```python
from build123d import *

# Parameters (mm, degrees)
SKETCH1_W                                       = 100
SKETCH1_H                                       = 28
BOSS_EXTRUDE1_DEPTH                             = 8
CSK_FOR_M6_FLAT_HEAD_MACHINE_SCREW1_D           = 6.6
CSK_FOR_M6_FLAT_HEAD_MACHINE_SCREW1_DEPTH       = 8
CSK_FOR_M6_FLAT_HEAD_MACHINE_SCREW1_CSINK_D     = 12.6
CSK_FOR_M6_FLAT_HEAD_MACHINE_SCREW1_CSINK_ANGLE = 90


with BuildPart() as part:
    # Sketch1 → Boss-Extrude1 (new body)
    with BuildSketch(Plane(origin=(0, 0, 0), x_dir=(1, 0, 0), z_dir=(0, 1, 0))):
        Rectangle(SKETCH1_W, SKETCH1_H)
    extrude(amount=BOSS_EXTRUDE1_DEPTH)

    # CSK for M6 Flat Head Machine Screw1
    with Locations(Plane(origin=(0, 8, 0), x_dir=(-1, 0, 0), z_dir=(0, 1, 0))):
        with Locations((-30, 0), (30, 0)):
            CounterSinkHole(CSK_FOR_M6_FLAT_HEAD_MACHINE_SCREW1_D / 2, CSK_FOR_M6_FLAT_HEAD_MACHINE_SCREW1_CSINK_D / 2, depth=CSK_FOR_M6_FLAT_HEAD_MACHINE_SCREW1_DEPTH, counter_sink_angle=CSK_FOR_M6_FLAT_HEAD_MACHINE_SCREW1_CSINK_ANGLE)


solid = part.part
```
Here's how the part is built. I have some questions about the finished solid (model axes, mm). Round coordinates to 2 decimals unless told otherwise and drop trailing zeros. Write each loop counter-clockwise with the first axis right and the second up, starting at its lowest first coordinate (ties: lowest second). Pieces come first, ordered by that corner, then holes.
Q1. If we mould it in two halves opening along Z, with no side actions, what happens to faces 1 (the flat face through (-1, 8, 0)), 2 (the conical face through (-26.71, 5.15, 1.03)), 3 (the flat face through (-1, 4, 14))? For each: +Z half, -Z half, draft (parallel to the pull), parting line (faces both ways), or undercut.
Q2. If we section it at B-B on y = 6.75: Write out the boundary of the cut face in (x, z).
Q3. Please list where these lines run through material, in increasing order: probe 1 along X at (y, z) = (3.1, 0); probe 2 along Z at (x, y) = (30, 2.15); probe 3 along X at (y, z) = (7, 2.75).
Q4. Will these pins go through, and if not, where does the flat tip stop? P1, Ø4, axis at x = 30, z = 0, coming from the -Y side; P2, Ø7.5, axis at x = -30, z = 0, coming from the +Y side.
Q5. If we section it at C-C on z = 0: Write out the boundary of the cut face in (x, y), plus the area to 3 significant figures.
Q6. If we section it at A-A on x = 30: Write out the boundary of the cut face in (y, z).
Answer below:
1. face 1: draft
1. face 2: undercut
1. face 3: +Z half
2. outline: (-50, -14) - (50, -14) - (50, 14) - (-50, 14) - close; hole circle Ø10.1 at (-30, 0); hole circle Ø10.1 at (30, 0)
3. probe 1: x = -50 to -33.3, -26.7 to 26.7, 33.3 to 50
3. probe 2: z = -14 to -3.3, 3.3 to 14
3. probe 3: x = -50 to -34.53, -25.47 to 25.47, 34.53 to 50
4. P1: passes through
4. P2: stops at y = 5.45
5. outline: (-50, 0) - (-33.3, 0) - (-33.3, 5) - (-36.3, 8) - (-50, 8) - close; (-26.7, 0) - (26.7, 0) - (26.7, 5) - (23.7, 8) - (-23.7, 8) - (-26.7, 5) - close; (33.3, 0) - (50, 0) - (50, 8) - (36.3, 8) - (33.3, 5) - close
5. area: 676 mm2
6. outline: (0, -14) - (8, -14) - (8, -6.3) - (5, -3.3) - (0, -3.3) - close; (0, 3.3) - (5, 3.3) - (8, 6.3) - (8, 14) - (0, 14) - close
